from build123d import *

# Parameters (mm, degrees)
SKETCH1_R           = 1.6
BOSS_EXTRUDE1_DEPTH = 2


with BuildPart() as part:
    # Sketch1 → Boss-Extrude1 (new body)
    with BuildSketch(Plane.XY):
        with BuildLine():
            Line((115.05, 10), (115.05, 11.6))
            Line((115.05, 11.6), (121.05, 11.6))
            Line((121.05, 11.6), (121.05, 10))
            ThreePointArc((121.05, 10), (122.05, 9), (123.05, 10))
            Line((123.05, 10), (123.55, 10))
            Line((123.55, 10), (123.55, 0))
            Line((123.55, 0), (123.05, 0))
            ThreePointArc((123.05, 0), (122.05, 1), (121.05, 0))
            Line((121.05, 0), (121.05, -1.6))
            Line((121.05, -1.6), (115.05, -1.6))
            Line((115.05, -1.6), (115.05, 0))
            ThreePointArc((115.05, 0), (114.05, 1), (113.05, 0))
            Line((113.05, 0), (112.55, 0))
            Line((112.55, 0), (112.55, 10))
            Line((112.55, 10), (113.05, 10))
            ThreePointArc((113.05, 10), (114.05, 9), (115.05, 10))
        make_face()
        with Locations((118.05, 5)):
            Circle(SKETCH1_R, mode=Mode.SUBTRACT)
    extrude(amount=BOSS_EXTRUDE1_DEPTH)


solid = part.part
Geometry: final body of the model. Coordinates: model frame, mm. A direction names the side the tool comes from. Round coordinates to 2 decimals unless told otherwise and drop trailing zeros. Loops run counter-clockwise (first coordinate to the right, second up) from the corner with the lowest first, then second, coordinate; pieces in that order, holes last. Notation, with made-up numbers: (-4.5, 71.25) - (34.5, 71.25) arc R24 cw to (34.5, 91.25) - close; hole circle Ø3 at (-37.75, 3.5). An arc over 180 degrees is marked (long way). Write each question's results on one line, items separated by ' | '. Start each with the question number.
1) Mould query, pull axis Y, two halves, no side actions, for faces 1 (the face through (119.53, 4.39, 0.99)), 2 (the face through (118, -1.6, 1)), 3 (the face through (115.05, -1, 1)), 4 (the face through (122, 9, 1)). Classes: released by +Y, released by -Y, zero draft, split by the parting line, or undercut.
2) First-contact query: P1, Ø0.6, axis at x = 123.5, z = 0.5, coming from the -Y side; P2, Ø0.8, axis at y = 10.5, z = 1, coming from the -X side; P3, Ø0.8, axis at y = -0.5, z = 1, coming from the +X side. Flat tips, straight axial feed; report the tip coordinate or a pass-through.
3) Cut plane D-D on y = 9.75. Return loops of the section in (x, z), then the cut area to 3 significant figures.
4) Cut plane B-B on x = 118.05. Return loops of the section in (y, z).
5) Line query: probe 1 along Y at (x, z) = (118.05, 1.6); probe 2 along X at (y, z) = (9.25, 0.8); probe 3 along Y at (x, z) = (119.5, 1.4). Output: solid intervals per line, ascending. Write a range as [from, to].
6) Cut plane C-C on z = 1. Return loops of the section in (x, y), then the cut area to 3 significant figures.
7) Access query for faces 5 (the face through (121.05, 11, 1)), 6 (the face through (115.05, 11, 1)), 7 (the face through (121.05, -1, 1)). Directions: +Z, -Z, +X, -X, +Y, -Y. A direction counts if a zero-diameter tool reaches every point of the face in a straight line with its end or side. Return the directions, or none.
8) Cut plane A-A on y = 5. Return loops of the section in (x, z).
Verdict:
1) face 1: undercut | face 2: released by -Y | face 3: zero draft | face 4: released by +Y
2) P1: stops at y = 0 | P2: stops at x = 115.05 | P3: stops at x = 121.05
3) outline: (112.55, 0) - (113.08, 0) - (113.08, 2) - (112.55, 2) - close; (115.02, 0) - (121.08, 0) - (121.08, 2) - (115.02, 2) - close; (123.02, 0) - (123.55, 0) - (123.55, 2) - (123.02, 2) - close | area: 14.3 mm2
4) outline: (-1.6, 0) - (3.4, 0) - (3.4, 2) - (-1.6, 2) - close; (6.6, 0) - (11.6, 0) - (11.6, 2) - (6.6, 2) - close
5) probe 1: y = [-1.6, 3.4], [6.6, 11.6] | probe 2: x = [112.55, 113.39], [114.71, 121.39], [122.71, 123.55] | probe 3: y = [-1.6, 4.32], [5.68, 11.6]
6) outline: (112.55, 0) - (113.05, 0) arc R1 cw to (115.05, 0) - (115.05, -1.6) - (121.05, -1.6) - (121.05, 0) arc R1 cw to (123.05, 0) - (123.55, 0) - (123.55, 10) - (123.05, 10) arc R1 cw to (121.05, 10) - (121.05, 11.6) - (115.05, 11.6) - (115.05, 10) arc R1 cw to (113.05, 10) - (112.55, 10) - close; hole circle Ø3.2 at (118.05, 5) | area: 115 mm2
7) face 5: +Z, -Z, +X, +Y | face 6: +Z, -Z, -X, +Y | face 7: +Z, -Z, +X, -Y
8) outline: (112.55, 0) - (116.45, 0) - (116.45, 2) - (112.55, 2) - close; (119.65, 0) - (123.55, 0) - (123.55, 2) - (119.65, 2) - close
